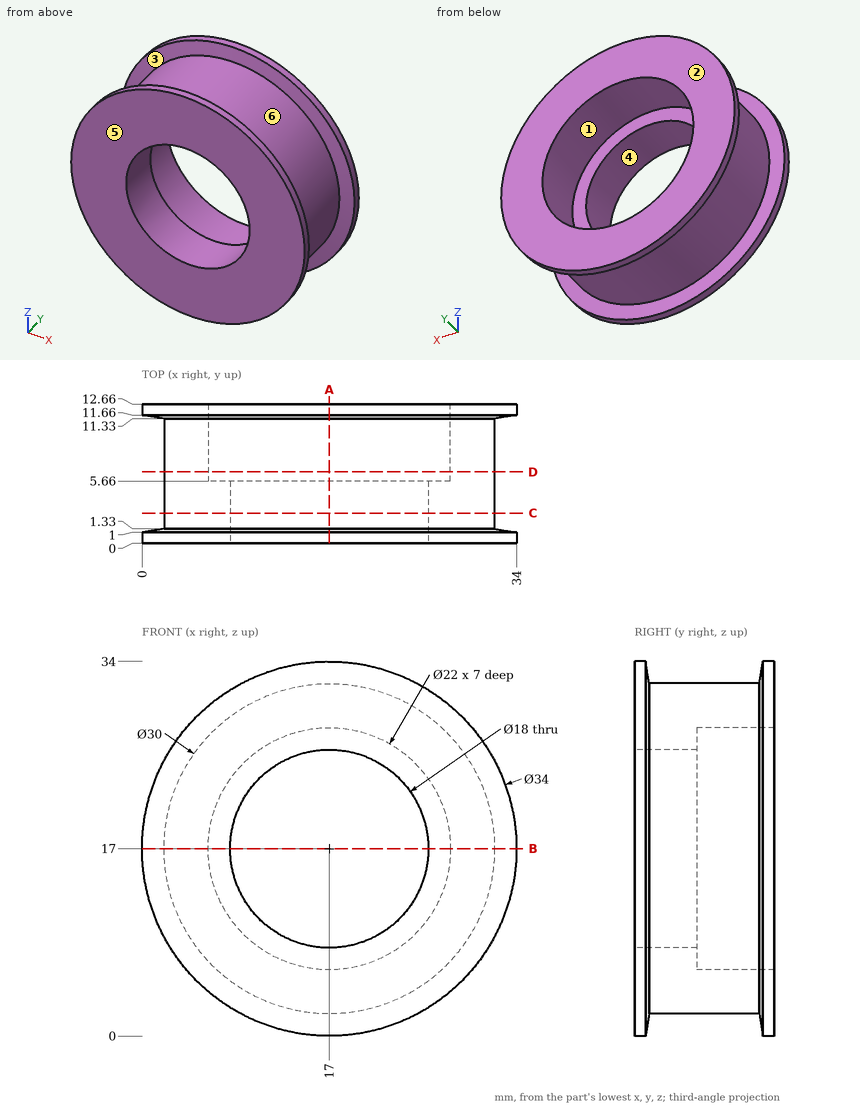
Job drawing, mm, ordinate dimensions from the low corner. One solid piece. A direction names the side the tool comes from. Coordinates: 2 decimals unless noted, no trailing zeros. Write each loop counter-clockwise with the first axis right and the second up, starting at its lowest first coordinate (ties: lowest second). Pieces come first, ordered by that corner, then holes. Notation, with made-up numbers: (60.5, 12) - (119.5, 12) arc R21 cw to (119.5, 31) - close; hole circle Ø9 at (-6.5, 6.25). An arc over 180 degrees is marked (long way). Use a Markdown table: item, result. Add a question column.
Item 1: Mould opens along Z. For the marked faces 4, 5 and 6 say: pulls with the +Z half, pulls with the -Z half, needs draft (parallel to the pull), parting line crosses it, or undercut.
Item 2: Band-saw the part on A-A, the plane x = 17. Give the cut face in (y, z), and give its area (3 significant figures).
Item 3: Drill centre lines: L1, parallel to X at y = 1.75, z = 17; L2, parallel to X at y = 8, z = 17. Where is each one in solid material? Low to high. Write a range as from..to.
Item 4: 3-axis set-ups, long thin cutter, end or side, ignore diameter. For the marked faces 1, 2 and 3: which of +Z, -Z, +X, -X, +Y, -Y reach the whole face in a straight line?
Item 5: Flat gauge pins, fed straight in: pin 1 (2 mm diameter, centred on y = 6.5, z = 13.5, fed in from -X); pin 2 (5 mm diameter, centred on x = 28, y = 7.5, fed in from +Z); pin 3 (6.5 mm diameter, centred on x = 14.5, z = 22, fed in from +Y); pin 4 (5 mm diameter, centred on y = 9.5, z = 23.5, fed in from -X). Where does each tip first touch, or does it go through?
Item 6: Band-saw the part on B-B, the plane z = 17. Give the cut face in (x, y).
Item 7: Band-saw the part on D-D, the plane y = 6.5. Give the cut face in (x, z), and give its area (3 significant figures).
Item 8: Band-saw the part on C-C, the plane y = 2.75. Give the cut face in (x, z), and give its area (3 significant figures).
Numbers:
| question | item | result |
|---|---|---|
| 1 | face 4 | undercut |
| 1 | face 5 | needs draft |
| 1 | face 6 | parting line crosses it |
| 2 | outline | (0, 0) - (1, 0) - (1.33, 2) - (11.33, 2) - (11.66, 0) - (12.66, 0) - (12.66, 6) - (5.66, 6) - (5.66, 8) - (0, 8) - close; (0, 26) - (5.66, 26) - (5.66, 28) - (12.66, 28) - (12.66, 34) - (11.66, 34) - (11.33, 32) - (1.33, 32) - (1, 34) - (0, 34) - close |
| 2 | area | 133 mm2 |
| 3 | L1 | 2..8, 26..32 |
| 3 | L2 | 2..6, 28..32 |
| 4 | face 1 | +Y |
| 4 | face 2 | +Z, -Z, +X, -X, +Y |
| 4 | face 3 | none |
| 5 | pin 1 | x = 2.21 |
| 5 | pin 2 | z = 29.36 |
| 5 | pin 3 | through |
| 5 | pin 4 | x = 0.83 |
| 6 | outline | (0, 0) - (8, 0) - (8, 5.66) - (6, 5.66) - (6, 12.66) - (0, 12.66) - (0, 11.66) - (2, 11.33) - (2, 1.33) - (0, 1) - close; (26, 0) - (34, 0) - (34, 1) - (32, 1.33) - (32, 11.33) - (34, 11.66) - (34, 12.66) - (28, 12.66) - (28, 5.66) - (26, 5.66) - close |
| 7 | outline | circle Ø30 at (17, 17); hole circle Ø22 at (17, 17) |
| 7 | area | 327 mm2 |
| 8 | outline | circle Ø30 at (17, 17); hole circle Ø18 at (17, 17) |
| 8 | area | 452 mm2 |
